Can you work these out from the model? Positions are in its coordinate system, mm. A direction names the side the tool comes from. Give positions to 0.01 mm unless a question says otherwise; leave off trailing zeros. Loops run counter-clockwise (first coordinate to the right, second up) from the corner with the lowest first, then second, coordinate; pieces in that order, holes last. Notation, with made-up numbers: (-27.75, 42.5) - (-21.75, 42.5) arc R10 cw to (-21.75, 50.5) - close; hole circle Ø5 at (52, 15.25). An arc over 180 degrees is marked (long way). Answer in a Markdown table with one row per item.
Autodesk Inventor part; units mm, degrees
ref_plane "YZ Plane" through (0, 0, 0) normal (1, 0, 0) x (0, 1, 0)
ref_plane "XZ Plane" through (0, 0, 0) normal (0, 1, 0) x (-1, 0, 0)
ref_plane "XY Plane" through (0, 0, 0) normal (0, 0, 1) x (1, 0, 0)
sketch "Sketch1" plane through (0, 0, 0) normal (0, 1, 0) x (-1, 0, 0)
  circle A0 centre (24.5, 0) radius 5.05
  circle A1 centre (39.5, 0) radius 5.05
  circle A2 centre (54.5, 0) radius 5.05
  circle A3 centre (69.5, 0) radius 5.05
  circle A4 centre (-69.5, 0) radius 5.05
  circle A5 centre (-54.5, 0) radius 5.05
  circle A6 centre (-39.5, 0) radius 5.05
  circle A7 centre (-24.5, 0) radius 5.05
  line L0 (69.5, -10) -> (11.1803, -10)
  line L1 (69.5, 10) -> (11.1803, 10)
  arc A8 (69.5, -10) -> (69.5, 10) centre (69.5, 0) ccw
  line L2 (-69.5, -10) -> (-11.1803, -10)
  arc A9 (-69.5, 10) -> (-69.5, -10) centre (-69.5, 0) ccw
  line L3 (-69.5, 10) -> (-11.1803, 10)
  arc A10 (11.1803, 10) -> (-11.1803, 10) centre (0, 0) ccw
  arc A11 (-11.1803, -10) -> (11.1803, -10) centre (0, 0) ccw
  dimension "d1" = 10.1
  dimension "d2" = 10.1
  dimension "d3" = 10.1
  dimension "d4" = 10.1
  dimension "d5" = 24.5
  dimension "d6" = 15
  dimension "d7" = 15
  dimension "d8" = 15
  dimension "d11" = 360
  dimension "d16" = 360
extrude "Extrusion1" add sketch "Sketch1" along normal blind 9
sketch "Sketch2" plane through (0, 0, 0) normal (0, -1, 0) x (1, 0, 0)
  circle A0 centre (-69.5, 0) radius 5.05
  circle A1 centre (-54.5, 0) radius 5.05
  circle A2 centre (-39.5, 0) radius 5.05
  circle A3 centre (-24.5, 0) radius 5.05
  circle A4 centre (24.5, 0) radius 5.05
  circle A5 centre (39.5, 0) radius 5.05
  circle A6 centre (54.5, 0) radius 5.05
  circle A7 centre (69.5, 0) radius 5.05
  circle A8 centre (-69.5, 0) radius 5.6
  circle A9 centre (-54.5, 0) radius 5.6
  circle A10 centre (-39.5, 0) radius 5.6
  circle A11 centre (-24.5, 0) radius 5.6
  circle A12 centre (24.5, 0) radius 5.6
  circle A13 centre (39.5, 0) radius 5.6
  circle A14 centre (54.5, 0) radius 5.6
  circle A15 centre (69.5, 0) radius 5.6
  point P0 (0, 0)
  dimension "d20" = 11.2
  dimension "d21" = 11.2
  dimension "d22" = 11.2
  dimension "d23" = 11.2
  dimension "d24" = 11.2
  dimension "d25" = 11.2
  dimension "d26" = 11.2
  dimension "d27" = 11.2
extrude "Extrusion2" cut sketch "Sketch2" against normal blind 2
sketch "Sketch5" plane through (0, 0, 0) normal (0, -1, 0) x (1, 0, 0)
  line L0 (9.9999, 7.45) -> (18.4999, 7.45)
  line L1 (18.4999, 7.45) -> (18.4999, -7.45)
  line L2 (18.4999, -7.45) -> (9.9999, -7.45)
  line L3 (9.9999, -7.45) -> (9.9999, 7.45)
  line L4 (69.5, 10) -> (11.1803, 10)
  circle A0 centre (14.1999, -4.5) radius 1.55
  point P0 (0, 0)
  point P1 (9.7499, -0.0369)
  dimension "d52" = 8.5
  dimension "d53" = 14.9
  dimension "d54" = 2.55
  dimension "d55" = 0.25
  dimension "d56" = 3.1
  dimension "d57" = 2.95
extrude "Extrusion4" cut sketch "Sketch5" against normal blind 3.5
sketch "Sketch6" plane through (0, 0, 0) normal (0, -1, 0) x (1, 0, 0)
  circle A0 centre (32, 6) radius 2
  circle A1 centre (24.5, 0) radius 5.05
  circle A2 centre (-32, -6) radius 2
  circle A3 centre (-24.5, 0) radius 5.05
  point P0 (0, 0)
  dimension "d60" = 4
  dimension "d61" = 7.5
  dimension "d62" = 6
  dimension "d63" = 4
  dimension "d64" = 7.5
  dimension "d65" = 6
extrude "Extrusion5" cut sketch "Sketch6" against normal through all contours A0 | A2
sketch "Sketch8" plane through (0, 0, 0) normal (0, -1, 0) x (1, 0, 0)
  point P0 (0, 0)
  point P1 (0, 0)
ref_plane "Work Plane1" through (-0.0001, 0, 7.45) normal (1, 0, 0) x (0, 0, -1)
sketch "Sketch9" plane through (-0.0001, 0, 7.45) normal (1, 0, 0) x (0, 0, -1)
  line L0 (7.45, 0) -> (-2.3, 0)
  line L1 (-2.55, 0) -> (17.45, 0)
  line L2 (7.45, 0) -> (7.45, -9)
  line L3 (7.45, -9) -> (-2.3, -9)
  line L4 (-2.3, -9) -> (0.45, -4.5)
  line L5 (-2.3, 0) -> (0.45, -4.5)
  dimension "d74" = 9
revolve "Revolution1" add sketch "Sketch9" angle 360 about axis through (-0.0001, 0, 0) along (0, -1, 0)
sketch "Sketch10" plane through (-0.0001, -9, 0) normal (0, -1, 0) x (1, 0, 0)
  circle A0 centre (0.0001, 0) radius 4.1
  dimension "d76" = 8.2
extrude "Extrusion6" cut sketch "Sketch10" against normal through all
chamfer "Chamfer1" distance 1 angle 45 1 edges at (-0.0001, -9, -9.75)
properties part number "led-prop"
Q1. If I drill on line 1 (Z direction, x = -54.5, y = 0.85); line 2 (Z direction, x = -54.5, y = 4.5); line 3 (Y direction, x = -65.5, z = 9.5), over which ranges is the centre line in solid material (lowest first)? Write a range as [from, to].
Checked values:
| item | result |
|---|---|
| line 1 | z = [-10, -5.6], [5.6, 10] |
| line 2 | z = [-10, -5.05], [5.05, 10] |
| line 3 | y = [0, 9] |
Q2. For pin 1 (5.5 mm diameter, centred on x = 69, z = -2, fed in from -Y); pin 2 (5 mm diameter, centred on x = 32, z = 6, fed in from -Y); pin 3 (8 mm diameter, centred on y = -2.5, z = -3.5, fed in from +X); pin 4 (3 mm diameter, centred on x = 23, y = 2.5, fed in from -Z), each with a flat end and sliding along its axis, tell me the tip position at first contact or that it passes through.
Checked values:
| item | result |
|---|---|
| pin 1 | passes through |
| pin 2 | stops at y = 0 |
| pin 3 | stops at x = 79.49 |
| pin 4 | stops at z = -10 |
Q3. Imagine slicing it at C-C, the plane y = -1.75. Write out the boundary of the cut face in (x, z), and give its area (3 significant figures).
Checked values:
| item | result |
|---|---|
| outline | circle Ø17.36 at (0, 0); hole circle Ø8.2 at (0, 0) |
| area | 184 mm² |
Q4. Imagine slicing it at B-B, the plane x = -39.5. Write out the boundary of the cut face in (y, z).
Checked values:
| item | result |
|---|---|
| outline | (0, -10) - (9, -10) - (9, -5.05) - (2, -5.05) - (2, -5.6) - (0, -5.6) - close; (0, 5.6) - (2, 5.6) - (2, 5.05) - (9, 5.05) - (9, 10) - (0, 10) - close |
Q5. On a 3-axis mill with a long thin cutter (end or side, diameter ignored), from which of +Z, -Z, +X, -X, +Y, -Y can I reach the whole of each face in a straight line? I mean faces 1 (the face through (14, 0, -4)), 2 (the face through (-41, 4, -10)), 3 (the face through (-74, 2, 3)). Say none if no direction works.
Checked values:
| item | result |
|---|---|
| face 1 | +Z, -Z, +X, -Y |
| face 2 | -Z, -X, +Y, -Y |
| face 3 | -Y |
Q6. If we mould it in two halves opening along X, with no side actions, what happens to faces 4 (the face through (0, 4, 15)), 5 (the face through (1, 9, -6)), 6 (the face through (-60.095, 0.986, 0.246))? For each: released by +X, released by -X, zero draft, split by the parting line, or undercut.
Checked values:
| item | result |
|---|---|
| face 4 | split by the parting line |
| face 5 | zero draft |
| face 6 | undercut |
Q7. Imagine slicing it at A-A, the plane y = 6.5. Count the separate pieces of the cut face and the enclosed holes in it, and give its area (3 significant figures).
Checked values:
| item | result |
|---|---|
| separate pieces | 1 |
| enclosed holes | 11 |
| area | 2,530 mm² |
